Work out the finished part from the listing and answer in its coordinate system (mm). A direction names the side the tool comes from. Give positions to 0.01 mm unless a question says otherwise; leave off trailing zeros. Write each loop counter-clockwise with the first axis right and the second up, starting at its lowest first coordinate (ties: lowest second). Pieces come first, ordered by that corner, then holes.
1) Given pin 1 Ø10 at (x, z) = (4.5, 23.5) entering from -Y; pin 2 Ø8 at (y, z) = (6.5, 28.5) entering from -X; pin 3 Ø1.5 at (y, z) = (0, 41) entering from -X; pin 4 Ø3.5 at (x, y) = (0, 0) entering from +Z, each flat-ended and moving along its own axis, determine where each tip first touches the part or whether it passes through.
2) Find section D-D (x = -7.5). Determine the outline of the cut face in (y, z), plus the area to 3 significant figures.
3) A tool of negligible diameter and unlimited length cuts with its end or side. For faces 4 (the face through (2, 0, 6)), 5 (the face through (-5.34, -0.05, 6.23)), 6 (the face through (0, -2, 45)), 7 (the face through (1.55, 0.34, 40.94)), from which of +Z, -Z, +X, -X, +Y, -Y can it reach the whole face along a straight path? Write none if from no direction.
4) Straight lines are drawn through the part: probe 1 along Z at (x, y) = (-6, 0); probe 2 along Y at (x, z) = (0, 41); probe 3 along Z at (x, y) = (-3, -1). For each, find the intervals that lie inside material, in ascending order.
5) Determine the mould class of faces 1 (the face through (-6.633, -6.083, 22.185)), 2 (the face through (-0.27, 0.06, 36.21)), 3 (the face through (-7.34, -0.091, 26.065)) for opening direction X: pulls with the +X half, pulls with the -X half, needs draft (parallel to the pull), parting line crosses it, or undercut.
6) Find section C-C (y = 7.25). Determine the outline of the cut face in (x, z), plus the area to 3 significant figures.
7) Find section B-B (z = 24). Determine the outline of the cut face in (x, y).
8) Find section A-A (x = 4). Determine the outline of the cut face in (y, z), plus the area to 3 significant figures.
Autodesk Inventor part; units mm, degrees
ref_plane "YZ Plane" through (0, 0, 0) normal (1, 0, 0) x (0, 1, 0)
ref_plane "XZ Plane" through (0, 0, 0) normal (0, 1, 0) x (-1, 0, 0)
ref_plane "XY Plane" through (0, 0, 0) normal (0, 0, 1) x (1, 0, 0)
sketch "Sketch1" plane through (0, 0, 0) normal (0, 0, 1) x (1, 0, 0)
  circle A0 centre (0, 0) radius 9
  dimension "d0" = 18
extrude "Extrusion1" add sketch "Sketch1" along normal blind 45
sketch "Sketch2" plane through (0, 0, 45) normal (0, 0, 1) x (1, 0, 0)
  point P0 (0, 0)
  point P1 (0, 0)
hole "Hole1" at (0, 0, 45) direction (0, 0, -1) diameter 3.175 depth 8 tip angle 118
sketch "Sketch3" plane through (0, 0, 0) normal (0, 0, -1) x (-1, 0, 0)
  point P0 (0, 0)
  point P1 (0, 0)
hole "Hole2" at (0, 0, 0) direction (0, 0, 1) diameter 4 depth 12 tip angle 118
sketch "Sketch4" plane through (0, 0, 0) normal (0, 1, 0) x (-1, 0, 0)
  circle A0 centre (0, 24) radius 6
  line L0 (9, 45) -> (-9, 45)
  point P0 (0, 0)
  dimension "d17" = 21
  dimension "d18" = 12
extrude "Extrusion2" cut sketch "Sketch4" along normal through all both and the other way through all
sketch "Sketch5" plane through (0, 0, 0) normal (1, 0, 0) x (0, 1, 0)
  line L0 (9, 45) -> (-9, 45)
  line L1 (-9, 0) -> (9, 0)
  point P0 (0, 0)
  point P1 (0, 41)
  point P2 (0, 5)
  dimension "d21" = 4
  dimension "d22" = 5
hole "Hole3" at (0, 0, 41) at (0, 0, 5) direction (-1, 0, 0) diameter 2.459 end through all
sketch "Sketch6" plane through (0, 0, 0) normal (1, 0, 0) x (0, 1, 0)
  line L0 (-9, 0) -> (9, 0)
  point P0 (0, 0)
  point P1 (0, 24)
  dimension "d30" = 24
hole "Hole4" at (0, 0, 24) direction (-1, 0, 0) diameter 4.134 end through all
properties part number "MotorPotCouple"
Results:
1. pin 1: stops at y = -8.51
1. pin 2: stops at x = -8.65
1. pin 3: stops at x = 1.4
1. pin 4: stops at z = 45
2. outline: (-4.97, 0) - (4.97, 0) - (4.97, 45) - (-4.97, 45) - close; hole circle Ø4.13 at (0, 24); hole circle Ø2.46 at (0, 5); hole circle Ø2.46 at (0, 41)
2. area: 425 mm2
3. face 4: -Z
3. face 5: -X
3. face 6: +Z, +X, -X, +Y, -Y
3. face 7: +Z
4. probe 1: z = 0 to 3.77, 6.23 to 21.93, 26.07 to 39.77, 42.23 to 45
4. probe 2: y = -9 to -1.59, 1.59 to 9
4. probe 3: z = 0 to 4.28, 5.72 to 18.8, 29.2 to 40.28, 41.72 to 45
5. face 1: parting line crosses it
5. face 2: undercut
5. face 3: needs draft
6. outline: (-5.33, 0) - (5.33, 0) - (5.33, 21.25) arc R6 cw to (-5.33, 21.25) - close; (-5.33, 26.75) arc R6 cw to (5.33, 26.75) - (5.33, 45) - (-5.33, 45) - close
6. area: 372 mm2
7. outline: (-8.76, -2.07) arc R9 ccw to (-6, -6.71) - (-6, -2.07) - close; (-8.76, 2.07) - (-6, 2.07) - (-6, 6.71) arc R9 ccw to start; (6, -6.71) arc R9 ccw to (6, 6.71) - close
8. outline: (-8.06, 0) - (8.06, 0) - (8.06, 19.53) - (-8.06, 19.53) - close; (-8.06, 28.47) - (8.06, 28.47) - (8.06, 45) - (-8.06, 45) - close
8. area: 581 mm2
